from build123d import *

# Parameters (mm, degrees)
F0_R     = 1.6
F1_DEPTH = 5


with BuildPart() as f1:
    # F0 (on Top) → F1 (new body)
    with BuildSketch(Plane.XY):
        with BuildLine():
            Line((0, -23.710678), (0, 0))
            Line((0, 0), (-15, 0))
            Line((-15, 0), (-15, -5))
            Line((-15, -5), (-28, -5))
            Line((-28, -5), (-28, -8.5))
            ThreePointArc((-28, -8.5), (-25.101021, -10.692753), (-24, -14.156854))
            Line((-24, -14.156854), (-24, -19.156854))
            Line((-24, -19.156854), (-36, -19.156854))
            Line((-36, -19.156854), (-36, -14.156854))
            ThreePointArc((-36, -14.156854), (-34.898979, -10.692753), (-32, -8.5))
            Line((-32, -8.5), (-32, -5))
            Line((-32, -5), (-45, -5))
            Line((-45, -5), (-45, 0))
            Line((-45, 0), (-84.289322, 0))
            Line((-84.289322, 0), (-84.289322, -5))
            Line((-84.289322, -5), (-97.289322, -5))
            Line((-97.289322, -5), (-97.289322, -8.5))
            ThreePointArc((-97.289322, -8.5), (-94.390342, -10.692753), (-93.289322, -14.156854))
            Line((-93.289322, -14.156854), (-93.289322, -19.156854))
            Line((-93.289322, -19.156854), (-105.289322, -19.156854))
            Line((-105.289322, -19.156854), (-105.289322, -14.156854))
            ThreePointArc((-105.289322, -14.156854), (-104.188301, -10.692753), (-101.289322, -8.5))
            Line((-101.289322, -8.5), (-101.289322, -5))
            Line((-101.289322, -5), (-114.289322, -5))
            Line((-114.289322, -5), (-114.289322, 0))
            Line((-114.289322, 0), (-124.289322, 0))
            Line((-124.289322, 0), (-131.36039, -7.071068))
            Line((-131.36039, -7.071068), (-134.895924, -3.535534))
            Line((-134.895924, -3.535534), (-156.109127, -24.748737))
            Line((-156.109127, -24.748737), (-152.573593, -28.284271))
            Line((-152.573593, -28.284271), (-172.372583, -48.083261))
            Line((-172.372583, -48.083261), (-169.897709, -50.558135))
            ThreePointArc((-169.897709, -50.558135), (-166.297311, -50.058757), (-163.069282, -51.729708))
            Line((-163.069282, -51.729708), (-159.533748, -55.265242))
            Line((-159.533748, -55.265242), (-168.01903, -63.750523))
            Line((-168.01903, -63.750523), (-171.554564, -60.214989))
            ThreePointArc((-171.554564, -60.214989), (-173.225514, -56.98696), (-172.726136, -53.386562))
            Line((-172.726136, -53.386562), (-175.20101, -50.911688))
            Line((-175.20101, -50.911688), (-195, -70.710678))
            Line((-195, -70.710678), (-170, -70.710678))
            Line((-170, -70.710678), (-170, -75.710678))
            Line((-170, -75.710678), (-140, -75.710678))
            Line((-140, -75.710678), (-140, -70.710678))
            Line((-140, -70.710678), (-55, -70.710678))
            Line((-55, -70.710678), (-55, -75.710678))
            Line((-55, -75.710678), (-25, -75.710678))
            Line((-25, -75.710678), (-25, -70.710678))
            Line((-25, -70.710678), (0, -70.710678))
            Line((0, -70.710678), (0, -53.710678))
            Line((0, -53.710678), (-5, -53.710678))
            Line((-5, -53.710678), (-5, -40.710678))
            Line((-5, -40.710678), (-8.5, -40.710678))
            ThreePointArc((-8.5, -40.710678), (-10.692753, -43.609658), (-14.156854, -44.710678))
            Line((-14.156854, -44.710678), (-19.156854, -44.710678))
            Line((-19.156854, -44.710678), (-19.156854, -32.710678))
            Line((-19.156854, -32.710678), (-14.156854, -32.710678))
            ThreePointArc((-14.156854, -32.710678), (-10.692753, -33.811699), (-8.5, -36.710678))
            Line((-8.5, -36.710678), (-5, -36.710678))
            Line((-5, -36.710678), (-5, -23.710678))
            Line((-5, -23.710678), (0, -23.710678))
        make_face()
        with Locations((-155, -73.210678)):
            Circle(F0_R, mode=Mode.SUBTRACT)
        with BuildLine():
            ThreePointArc((-125, -58.210678), (-124.267767, -56.442911), (-122.5, -55.710678))
            Line((-122.5, -55.710678), (-52.5, -55.710678))
            ThreePointArc((-52.5, -55.710678), (-50.732233, -56.442911), (-50, -58.210678))
            ThreePointArc((-50, -58.210678), (-50.732233, -59.978445), (-52.5, -60.710678))
            Line((-52.5, -60.710678), (-122.5, -60.710678))
            ThreePointArc((-122.5, -60.710678), (-124.267767, -59.978445), (-125, -58.210678))
        make_face(mode=Mode.SUBTRACT)
        with Locations((-40, -73.210678)):
            Circle(F0_R, mode=Mode.SUBTRACT)
        with BuildLine():
            ThreePointArc((-125, -48.210678), (-124.267767, -46.442911), (-122.5, -45.710678))
            Line((-122.5, -45.710678), (-52.5, -45.710678))
            ThreePointArc((-52.5, -45.710678), (-50.732233, -46.442911), (-50, -48.210678))
            ThreePointArc((-50, -48.210678), (-50.732233, -49.978445), (-52.5, -50.710678))
            Line((-52.5, -50.710678), (-122.5, -50.710678))
            ThreePointArc((-122.5, -50.710678), (-124.267767, -49.978445), (-125, -48.210678))
        make_face(mode=Mode.SUBTRACT)
        with BuildLine():
            ThreePointArc((-125, -38.210678), (-124.267767, -36.442911), (-122.5, -35.710678))
            Line((-122.5, -35.710678), (-52.5, -35.710678))
            ThreePointArc((-52.5, -35.710678), (-50.732233, -36.442911), (-50, -38.210678))
            ThreePointArc((-50, -38.210678), (-50.732233, -39.978445), (-52.5, -40.710678))
            Line((-52.5, -40.710678), (-122.5, -40.710678))
            ThreePointArc((-122.5, -40.710678), (-124.267767, -39.978445), (-125, -38.210678))
        make_face(mode=Mode.SUBTRACT)
        with Locations((-143.734758, -15.909903)):
            Circle(F0_R, mode=Mode.SUBTRACT)
    extrude(amount=F1_DEPTH)


solid = f1.part
Verification items for the finished model (mm, model axes). A direction names the side the tool comes from. Give positions to 0.01 mm unless a question says otherwise; leave off trailing zeros. Write each loop counter-clockwise with the first axis right and the second up, starting at its lowest first coordinate (ties: lowest second). Pieces come first, ordered by that corner, then holes. Notation, with made-up numbers: (9.5, 1) -> (45.5, 1) arc R28 cw to (45.5, 29) -> close; hole circle Ø9 at (-38, 69.25). An arc over 180 degrees is marked (long way). Use CSV: the item, a comma, the result in double quotes.
(1) Sectioned sample at C-C (z = 2.35). Give the number of separate pieces and of enclosed holes in the cut face, plus the area to 3 significant figures.
Derived:
separate pieces,"1"
enclosed holes,"6"
area,"9,640 mm^2"
(2) Release check for a two-part mould opening along Y. For faces 6 (the flat face through (-183, -70.711, 2)), 7 (the flat face through (-15, -2, 2)), 8 (the flat face through (-36, -17, 2)) record: +Y half, -Y half, draft (parallel to the pull), parting line (faces both ways), or undercut.
Derived:
face 6,"-Y half"
face 7,"draft"
face 8,"undercut"
(3) Sectioned sample at B-B (y = -30.5). Record the cut outline in (x, z), plus the area to 3 significant figures.
Derived:
outline,"(-154.79, 0) -> (-5, 0) -> (-5, 5) -> (-154.79, 5) -> close"
area,"749 mm^2"
(4) Go/stop test with flat-tipped pins: pin 1 (4 mm diameter, centred on x = -143.73, y = -15.91, fed in from +Z); pin 2 (3 mm diameter, centred on y = -29.5, z = 1.5, fed in from +X); pin 3 (1.8 mm diameter, centred on y = -7, z = 3.5, fed in from -X); pin 4 (1.5 mm diameter, centred on x = -90.5, z = 1.5, fed in from -Y). Record where each tip stops, or that it passes through.
Derived:
pin 1,"stops at z = 5"
pin 2,"stops at x = -5"
pin 3,"stops at x = -139.26"
pin 4,"stops at y = -70.71"
(5) Set-up check for faces 1 (the cylindrical face through (-166.35, -50.05, 2.46)), 2 (the flat face through (-38, -5, 2)), 3 (the flat face through (-13, -70.711, 2)), 4 (the flat face through (-7, -40.711, 2)), 5 (the flat face through (-119, 0, 2)): record each of +Z, -Z, +X, -X, +Y, -Y from which the full face is reachable in a straight line by a thin tool's end or side.
Derived:
face 1,"+Z, -Z"
face 2,"+Z, -Z, +Y"
face 3,"+Z, -Z, +X, -Y"
face 4,"+Z, -Z, +X"
face 5,"+Z, -Z, +X, -X, +Y"
(6) Sectioned sample at A-A (x = -118.5). Record the cut outline in (y, z), plus the area to 3 significant figures.
Derived:
outline,"(-70.71, 0) -> (-60.71, 0) -> (-60.71, 5) -> (-70.71, 5) -> close; (-55.71, 0) -> (-50.71, 0) -> (-50.71, 5) -> (-55.71, 5) -> close; (-45.71, 0) -> (-40.71, 0) -> (-40.71, 5) -> (-45.71, 5) -> close; (-35.71, 0) -> (0, 0) -> (0, 5) -> (-35.71, 5) -> close"
area,"279 mm^2"
(7) Material ranges on L1, parallel to Y at x = -81.5, z = 4.3; L2, parallel to X at y = -17, z = 3.8; L3, parallel to X at y = -9, z = 0.75, recorded low to high.
Derived:
L1,"y = -70.71 to -60.71, -55.71 to -50.71, -45.71 to -40.71, -35.71 to 0"
L2,"x = -148.36 to -144.91, -142.56 to -105.29, -93.29 to -36, -24 to 0"
L3,"x = -140.36 to -102.36, -96.22 to -33.07, -26.93 to 0"
